Check sheet for the modelled part. Datum: model origin and axes. Units: mm. A direction names the side the tool comes from. Give positions to 0.01 mm unless a question says otherwise; leave off trailing zeros. Loops run counter-clockwise (first coordinate to the right, second up) from the corner with the lowest first, then second, coordinate; pieces in that order, holes last. Notation, with made-up numbers: M 32,81.5 L 60,81.5 A12 ccw 60,98.5 Z; hole C 21.25,59.5 d2. An arc over 180 degrees is marked long. Use one line per item in the form item = value.
from build123d import *

# Parameters (mm, degrees)
DODANIE_WYCI_GNI_CIE1_DEPTH = 14.5
OTW_R_12_0_12_1_D           = 12
OTW_R_12_0_12_1_DEPTH       = 20
OTW_R_12_0_12_1_TIP         = 3.605163714
DODANIE_WYCI_GNI_CIE2_DEPTH = 3
DODANIE_WYCI_GNI_CIE3_START = 3
DODANIE_WYCI_GNI_CIE3_DEPTH = 3
DODANIE_WYCI_GNI_CIE4_DEPTH = 3
SZKIC7_W                    = 20
SZKIC7_H                    = 20
DODANIE_WYCI_GNI_CIE5_DEPTH = 3
SZKIC8_W                    = 20
SZKIC8_H                    = 30
DODANIE_WYCI_GNI_CIE6_DEPTH = 3
SZKIC9_R                    = 2
WYTNIJ_WYCI_GNI_CIE1_DEPTH  = 8
SZKIC10_R                   = 4
DODANIE_WYCI_GNI_CIE7_DEPTH = 5
WYTNIJ_WYCI_GNI_CIE2_START  = -5
SZKIC13_R                   = 2
WYTNIJ_WYCI_GNI_CIE2_DEPTH  = 5
DODANIE_WYCI_GNI_CIE8_DEPTH = 3
SFAZOWANIE1_SIZE            = 0.5
SZKIC18_R                   = 5
DODANIE_WYCI_GNI_CIE9_DEPTH = 10
SFAZOWANIE2_SIZE            = 1


with BuildPart() as part:
    # Szkic1 → Dodanie-wyciągnięcie1 (new, symmetric)
    with BuildSketch(Plane.XY):
        with BuildLine():
            Line((-60, 0), (-85, 0))
            Line((-85, 0), (-85, -30.5))
            Line((-85, -30.5), (-85, -70))
            Line((-85, -70), (85, -70))
            Line((85, -70), (85, -30.5))
            Line((85, -30.5), (85, 0))
            Line((85, 0), (60, 0))
            ThreePointArc((60, 0), (0, -60), (-60, 0))
        make_face()
    extrude(amount=DODANIE_WYCI_GNI_CIE1_DEPTH, both=True)

    # Otwór Ø12.0 (12)1
    with Locations(Plane(origin=(0, 0, 0), x_dir=(1, 0, 0), z_dir=(0, 1, 0))):
        with Locations((-70, 0), (70, 0)):
            Hole(OTW_R_12_0_12_1_D / 2, depth=OTW_R_12_0_12_1_DEPTH)
            with Locations((0, 0, -(OTW_R_12_0_12_1_DEPTH + OTW_R_12_0_12_1_TIP / 2))):  # 118° drill point
                Cone(0, OTW_R_12_0_12_1_D / 2, OTW_R_12_0_12_1_TIP, mode=Mode.SUBTRACT)

    # Szkic4 → Dodanie-wyciągnięcie2 (add)
    with BuildSketch(Plane(origin=(0, 0, -14.5), x_dir=(-1, 0, 0), z_dir=(0, 0, -1))):
        with BuildLine():
            Line((-53, 0), (-85, 0))
            Line((-85, 0), (-85, -70))
            Line((-85, -70), (85, -70))
            Line((85, -70), (85, 0))
            Line((85, 0), (53, 0))
            ThreePointArc((53, 0), (0, -53), (-53, 0))
        make_face()
    extrude(amount=DODANIE_WYCI_GNI_CIE2_DEPTH)

    # Szkic5 → Dodanie-wyciągnięcie3 (add)
    with BuildSketch(Plane.XY.offset(14.5).offset(DODANIE_WYCI_GNI_CIE3_START)):
        with BuildLine():
            Line((-53, 0), (-85, 0))
            Line((-85, 0), (-85, -70))
            Line((-85, -70), (85, -70))
            Line((85, -70), (85, 0))
            Line((85, 0), (53, 0))
            ThreePointArc((53, 0), (0, -53), (-53, 0))
        make_face()
    extrude(amount=-DODANIE_WYCI_GNI_CIE3_DEPTH)

    # Szkic6 → Dodanie-wyciągnięcie4 (add)
    with BuildSketch(Plane(origin=(0, -70, 0), x_dir=(1, 0, 0), z_dir=(0, 1, 0))):
        Polygon((0, 17.5), (-10, 17.5), (-10, 62.5), (10, 62.5), (10, 17.5), align=None)
    extrude(amount=DODANIE_WYCI_GNI_CIE4_DEPTH)

    # Szkic7 → Dodanie-wyciągnięcie5 (add)
    with BuildSketch(Plane(origin=(0, 0, -62.5), x_dir=(-1, 0, 0), z_dir=(0, 0, -1))):
        with Locations((0, -77)):
            Rectangle(SZKIC7_W, SZKIC7_H)
    extrude(amount=DODANIE_WYCI_GNI_CIE5_DEPTH)

    # Szkic8 → Dodanie-wyciągnięcie6 (add)
    with BuildSketch(Plane.XZ.offset(87)):
        with Locations((0, -50.5)):
            Rectangle(SZKIC8_W, SZKIC8_H)
    extrude(amount=DODANIE_WYCI_GNI_CIE6_DEPTH)

    # Szkic9 → Wytnij-wyciągnięcie1 (cut)
    with BuildSketch(Plane.XZ.offset(90)):
        with Locations(Location((0, -40.997300871, 0), (0, 0, 270))):
            Circle(SZKIC9_R)
    extrude(amount=-WYTNIJ_WYCI_GNI_CIE1_DEPTH, mode=Mode.SUBTRACT)

    # Szkic10 → Dodanie-wyciągnięcie7 (add)
    with BuildSketch(Plane(origin=(0, -87, 0), x_dir=(1, 0, 0), z_dir=(0, 1, 0))):
        with Locations(Location((0, 40.997300871, 0), (0, 0, 90))):
            Circle(SZKIC10_R)
    extrude(amount=DODANIE_WYCI_GNI_CIE7_DEPTH)

    # Szkic13 → Wytnij-wyciągnięcie2 (cut)
    with BuildSketch(Plane(origin=(0, -82, 0), x_dir=(1, 0, 0), z_dir=(0, 1, 0)).offset(WYTNIJ_WYCI_GNI_CIE2_START)):
        with Locations(Location((0, 40.997300871, 0), (0, 0, 90))):
            Circle(SZKIC13_R)
    extrude(amount=WYTNIJ_WYCI_GNI_CIE2_DEPTH, mode=Mode.SUBTRACT)

    # Szkic14 → Dodanie-wyciągnięcie8 (add)
    with BuildSketch(Plane(origin=(0, -70, 0), x_dir=(1, 0, 0), z_dir=(0, 1, 0))):
        Polygon((3, -17.5), (-3, -17.5), (-3, -42.5), (0, -47.5), (3, -42.5), align=None)
    extrude(amount=DODANIE_WYCI_GNI_CIE8_DEPTH)

    # Sfazowanie1
    sfazowanie1_edges = [part.edges().sort_by_distance(p)[0] for p in [
        (1.5, -67, 45),
        (-1.5, -67, 45),
    ]]
    chamfer(sfazowanie1_edges, length=SFAZOWANIE1_SIZE)

    # Szkic18 → Dodanie-wyciągnięcie9 (add)
    with BuildSketch(Plane(origin=(0, -70, 0), x_dir=(-1, 0, 0), z_dir=(0, -1, 0))):
        with Locations(Location((0, 0, 0), (0, 0, 270))):
            Circle(SZKIC18_R)
    extrude(amount=DODANIE_WYCI_GNI_CIE9_DEPTH)

    # Sfazowanie2
    sfazowanie2_edges = [part.edges().sort_by_distance(p)[0] for p in [
        (0, -80, -5),
    ]]
    chamfer(sfazowanie2_edges, length=SFAZOWANIE2_SIZE)


solid = part.part
1) Section check A-A (z = -54). Record the cut outline in (x, y).
Evaluation:
outline = M -10,-90 L 10,-90 L 10,-87 L -10,-87 Z; M -10,-70 L 10,-70 L 10,-67 L -10,-67 Z
2) Section check D-D (y = -56). Record the cut outline in (x, z).
Evaluation:
outline = M -85,-17.5 L 85,-17.5 L 85,17.5 L -85,17.5 Z; hole M -21.54,-14.5 L 21.54,-14.5 L 21.54,14.5 L -21.54,14.5 Z
3) Release check for a two-part mould opening along Z. For faces 4 (the face through (-1, -58, 17.5)), 5 (the face through (-4, -54, -14.5)), 6 (the face through (-10, -69, -51)) record: pulls with the +Z half, pulls with the -Z half, needs draft (parallel to the pull), parting line crosses it, or undercut.
Evaluation:
face_4 = pulls with the +Z half
face_5 = undercut
face_6 = needs draft
4) Set-up check for faces 1 (the face through (0, -78, -62.5)), 2 (the face through (1, -82, -39)), 3 (the face through (76, -10, 0)): record each of +Z, -Z, +X, -X, +Y, -Y from which the full face is reachable in a straight line by a thin tool's end or side.
Evaluation:
face_1 = +X, -X
face_2 = +Z, +X, -X
face_3 = +Y
5) Section check B-B (y = -6.5). Record the cut outline in (x, z).
Evaluation:
outline = M -85,-17.5 L -52.6,-17.5 L -52.6,-14.5 L -59.65,-14.5 L -59.65,14.5 L -52.6,14.5 L -52.6,17.5 L -85,17.5 Z; M 52.6,-17.5 L 85,-17.5 L 85,17.5 L 52.6,17.5 L 52.6,14.5 L 59.65,14.5 L 59.65,-14.5 L 52.6,-14.5 Z; hole C -70,0 d12; hole C 70,0 d12
6) Scan lines: line 1 (Z direction, x = -70, y = -7); line 2 (Y direction, x = 7, z = -52); line 3 (Y direction, x = -0.5, z = -38.5). Record each from-to range of solid material in increasing order.
Evaluation:
line_1 = -17.5 to -6, 6 to 17.5
line_2 = -90 to -87, -70 to -67
line_3 = -90 to -82, -70 to -67
7) Depth check by flat-ended pin: pin 1 Ø7 at (y, z) = (-79.5, -41) entering from +X; pin 2 Ø8 at (y, z) = (-49.5, 23.5) entering from +X; pin 3 Ø1 at (x, y) = (-10.5, -54) entering from +Z; pin 4 Ø22 at (x, z) = (-4, -43.5) entering from +Y. Enter the tip coordinate at first touch or a pass-through.
Evaluation:
pin_1 = 4
pin_2 = through
pin_3 = 17.5
pin_4 = -67
8) Section check C-C (y = -46.5). Record the cut outline in (x, z), then the cut area to 3 significant figures.
Evaluation:
outline = M -85,-17.5 L -25.43,-17.5 L -25.43,-14.5 L -37.92,-14.5 L -37.92,14.5 L -25.43,14.5 L -25.43,17.5 L -85,17.5 Z; M 25.43,-17.5 L 85,-17.5 L 85,17.5 L 25.43,17.5 L 25.43,14.5 L 37.92,14.5 L 37.92,-14.5 L 25.43,-14.5 Z
area = 3,450 mm^2
